Input: part model. Units: mm. Frame: model coordinates. Face numbers are marked on the shaded views. A direction names the side the tool comes from. Coordinates: 2 decimals unless noted, no trailing zeros. Loops run counter-clockwise (first coordinate to the right, second up) from the corner with the lowest first, then second, coordinate; pieces in that order, holes last. Notation, with made-up numbers: (24, 67.5) -> (82, 67.5) arc R35 cw to (82, 103.5) -> close; hole circle Ø9 at (51.25, -31.5). An arc over 180 degrees is marked (long way). Put each result on its own line as item: value. Start each with the question number.
1) Set-up query: the marked faces 1 and 2. Return all of +Z, -Z, +X, -X, +Y, -Y with unobstructed straight access to the full face (end or side cutting, diameter ignored); none if empty.
2) Cut plane C-C (y = 2.25). Return the cut outline in (x, z).
3) Pull-direction query (Y, two-part tool) for the marked faces 3, 4 and 5; classes: pulls with the +Y half, pulls with the -Y half, needs draft (parallel to the pull), parting line crosses it, or undercut.
4) Cut plane D-D (y = 9). Return the cut outline in (x, z).
5) Cut plane B-B (z = -5). State how many separate pieces and enclosed holes the cut face has, plus the area to 3 significant figures.
6) Contact query for flat-ended pins moving along their axis: P1, Ø3, axis at x = 3, y = 11.5, coming from the -Z side; P2, Ø1.1, axis at x = 1.5, y = 12.5, coming from the +Z side; P3, Ø1.5, axis at y = 4, z = -8, coming from the -X side. Output: stop coordinate, or through.
7) Cut plane A-A (y = 0.25). Return the cut outline in (x, z).
8) Material intervals for L1, parallel to Y at x = 3.2, z = -4.25; L2, parallel to X at y = 10.8, z = -5; L3, parallel to Y at x = 1.2, z = -8, sorted ascending.
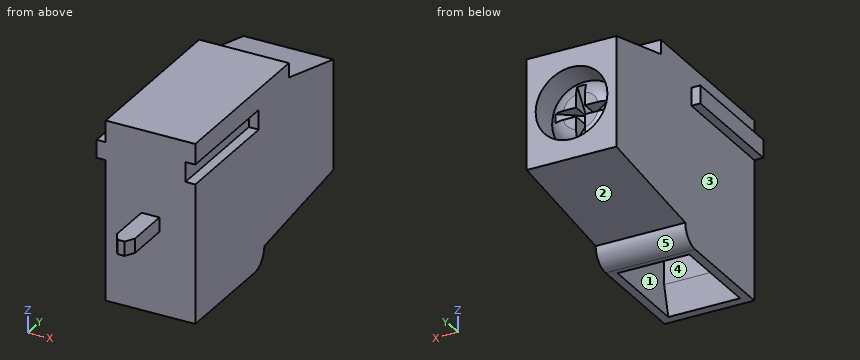
from build123d import *

# Parameters (mm, degrees)
BOSS_EXTRUDE1_DEPTH      = 5
CUT_EXTRUDE_1_DEPTH      = 4
SKETCH_4_R               = 2
CUT_EXTRUDE_2_DEPTH      = 4
CUT_EXTRUDE_START        = 0.25
CUT_EXTRUDE_3_DEPTH      = 0.5
PATTERN_CIRCULAR_2_COUNT = 4
SKETCH_7_W               = 1
SKETCH_7_H               = 6.38564687
EXTRUDE_1_DEPTH          = 0.5
SKETCH_8_W               = 1.1
SKETCH_8_H               = 6.43564687
CUT_EXTRUDE_4_DEPTH      = 0.55
SKETCH_10_W              = 1
SKETCH_10_H              = 0.8
EXTRUDE_2_DEPTH          = 3
CHAMFER_2_SIZE           = 0.3
CHAMFER_2_SIZE2          = 0.519615242
CHAMFER_3_SIZE           = 0.3
CHAMFER_3_SIZE2          = 0.519615242


with BuildPart() as part:
    # Sketch1 → Boss-Extrude1 (new body)
    with BuildSketch(Plane(origin=(0, 0, 0), x_dir=(0, 0, -1), z_dir=(1, 0, 0))):
        with BuildLine():
            Line((8.071293529, 14), (8.983255455, 7))
            Line((8.983255455, 7), (9, 7))
            ThreePointArc((9, 7), (9.707106781, 6.707106781), (10, 6))
            Line((10, 6), (10, 0))
            Line((10, 0), (0, 0))
            Line((0, 0), (0, 9.493570114))
            Line((0, 9.493570114), (0.802161187, 9.493570114))
            Line((0.802161187, 9.493570114), (1.928706471, 14))
            Line((1.928706471, 14), (8.071293529, 14))
        make_face()
    extrude(amount=BOSS_EXTRUDE1_DEPTH)

    # Sketch 2 → Cut-Extrude 1 (cut)
    with BuildSketch(Plane.ZY.offset(-0.5)):
        Polygon((-10, 5.692040605), (-8.656873738, 5.046895275), (-2.931105615, 5.046895275), (-2.931105615, 0.968562632), (-8.400228705, 0.968562632), (-10, 0.542354651), align=None)
    extrude(amount=-CUT_EXTRUDE_1_DEPTH, mode=Mode.SUBTRACT)

    # Sketch 4 → Cut-Extrude 2 (cut)
    with BuildSketch(Plane(origin=(0, 14, 0), x_dir=(1, 0, 0), z_dir=(0, 1, 0))):
        with Locations(Location((2.5, 5, 0), (0, 0, 270))):
            Circle(SKETCH_4_R)
    extrude(amount=-CUT_EXTRUDE_2_DEPTH, mode=Mode.SUBTRACT)

    # Sketch 5 → Revolve 1 (revolve)
    with BuildSketch(Plane.ZY.offset(-2.5), mode=Mode.PRIVATE) as revolve_1_sk:
        with BuildLine():
            Line((-5, 13.076817247), (-6, 13.076817247))
            ThreePointArc((-6, 13.076817247), (-6.707106781, 12.783924028), (-7, 12.076817247))
            Line((-7, 12.076817247), (-7, 11.356355107))
            Line((-7, 11.356355107), (-5, 11.356355107))
            Line((-5, 11.356355107), (-5, 13.076817247))
        make_face()
    revolve(revolve_1_sk.sketch.rotate(Axis((2.5, 13.076817247, -5), (0, -1, 0)), 180), axis=Axis((2.5, 13.076817247, -5), (0, -1, 0)))

    # Sketch 6 → Cut-Extrude 3 (cut)
    with BuildSketch(Plane.ZY.offset(-2.5).offset(CUT_EXTRUDE_START)):
        Polygon((-6.758727889, 13.191820369), (-5, 13.191820369), (-5, 12.042931868), (-5.25, 12.042931868), align=None)
    cut_extrude_3 = extrude(amount=-CUT_EXTRUDE_3_DEPTH, mode=Mode.SUBTRACT)

    # Pattern Circular 2: Cut-Extrude 3 ×4 about axis
    pattern_circular_2_axis = Axis((2.5, 0, -5), (0, 1, 0))
    for i in range(1, PATTERN_CIRCULAR_2_COUNT):
        add(cut_extrude_3.rotate(pattern_circular_2_axis, i * 360 / PATTERN_CIRCULAR_2_COUNT), mode=Mode.SUBTRACT)

    # Sketch 7 → Extrude 1 (add)
    with BuildSketch(Plane.ZY):
        with Locations((-1.7, 3.192823435)):
            Rectangle(SKETCH_7_W, SKETCH_7_H)
    extrude(amount=EXTRUDE_1_DEPTH)

    # Sketch 8 → Cut-Extrude 4 (cut)
    with BuildSketch(Plane(origin=(5, 0, 0), x_dir=(0, 0, -1), z_dir=(1, 0, 0))):
        with Locations((1.7, 3.217823435)):
            Rectangle(SKETCH_8_W, SKETCH_8_H)
    extrude(amount=-CUT_EXTRUDE_4_DEPTH, mode=Mode.SUBTRACT)

    # Sketch 10 → Extrude 2 (add)
    with BuildSketch(Plane(origin=(0, 0, 0), x_dir=(-1, 0, 0), z_dir=(0, -1, 0))):
        with Locations((-2.5, 5)):
            Rectangle(SKETCH_10_W, SKETCH_10_H)
    extrude(amount=EXTRUDE_2_DEPTH)

    # Chamfer 2
    chamfer_2_edges = [part.edges().sort_by_distance(p)[0] for p in [
        (2, -3, -5),
    ]]
    chamfer_2_side = [part.faces().sort_by_distance(p)[0] for p in [
        (2.5, -3, -5),
    ]]
    chamfer(chamfer_2_edges, length=CHAMFER_2_SIZE, length2=CHAMFER_2_SIZE2, reference=chamfer_2_side[0])

    # Chamfer 3
    chamfer_3_edges = [part.edges().sort_by_distance(p)[0] for p in [
        (3, -3, -5),
    ]]
    chamfer_3_side = [part.faces().sort_by_distance(p)[0] for p in [
        (2.65, -3, -5),
    ]]
    chamfer(chamfer_3_edges, length=CHAMFER_3_SIZE, length2=CHAMFER_3_SIZE2, reference=chamfer_3_side[0])


solid = part.part
Results found:
1. face 1: -Z
1. face 2: -Z, +X, -X, +Y
2. outline: (-0.5, -2.2) -> (0, -2.2) -> (0, -10) -> (0.5, -10) -> (0.5, -2.93) -> (4.5, -2.93) -> (4.5, -10) -> (5, -10) -> (5, -2.25) -> (4.45, -2.25) -> (4.45, -1.15) -> (5, -1.15) -> (5, 0) -> (0, 0) -> (0, -1.2) -> (-0.5, -1.2) -> close
3. face 3: needs draft
3. face 4: undercut
3. face 5: pulls with the +Y half
4. outline: (0, -8.72) -> (5, -8.72) -> (5, 0) -> (0, 0) -> close
5. separate pieces: 1
5. enclosed holes: 2
5. area: 45.1 mm2
6. P1: stops at z = -8.59
6. P2: stops at z = -1.42
6. P3: stops at x = 0
7. outline: (-0.5, -2.2) -> (0, -2.2) -> (0, -10) -> (5, -10) -> (5, -2.25) -> (4.45, -2.25) -> (4.45, -1.15) -> (5, -1.15) -> (5, 0) -> (0, 0) -> (0, -1.2) -> (-0.5, -1.2) -> close
8. L1: y = 0 to 0.97, 5.05 to 10, 11.36 to 13.08
8. L2: x = 0 to 0.5, 4.5 to 5
8. L3: y = 0 to 0.97, 5.05 to 14
